```python
from build123d import *

# Parameters (mm, degrees)
BOSS_EXTRUDE1_DEPTH = 76.2
SKETCH2_R           = 2.413
CUT_EXTRUDE1_DEPTH  = 3.175
SKETCH4_R           = 2.413
CUT_EXTRUDE2_DEPTH  = 104.224128115


with BuildPart() as part:
    # Sketch1 → Boss-Extrude1 (new body)
    with BuildSketch(Plane(origin=(0, 0, 0), x_dir=(1, 0, 0), z_dir=(0, 1, 0))):
        Polygon((0, 50.8), (0, 0), (50.8, 0), (50.8, 3.175), (3.175, 3.175), (3.175, 50.8), align=None)
    extrude(amount=BOSS_EXTRUDE1_DEPTH)

    # Sketch2 → Cut-Extrude1 (cut)
    with BuildSketch(Plane(origin=(0, 0, -3.175), x_dir=(-1, 0, 0), z_dir=(0, 0, -1))):
        Polygon((-50.8, 12.7188211), (-6.35, 76.2), (-50.8, 76.2), align=None)
        with Locations((-13.335, 6.35)):
            Circle(SKETCH2_R)
        with Locations((-26.035, 6.35)):
            Circle(SKETCH2_R)
        with Locations((-13.335, 19.05)):
            Circle(SKETCH2_R)
        with Locations((-13.335, 31.75)):
            Circle(SKETCH2_R)
        with Locations((-13.335, 44.45)):
            Circle(SKETCH2_R)
        with Locations((-26.035, 19.05)):
            Circle(SKETCH2_R)
        with Locations((-26.035, 31.75)):
            Circle(SKETCH2_R)
        with Locations((-38.735, 19.05)):
            Circle(SKETCH2_R)
        with Locations((-38.735, 6.35)):
            Circle(SKETCH2_R)
    extrude(amount=-CUT_EXTRUDE1_DEPTH, mode=Mode.SUBTRACT)

    # Sketch4 → Cut-Extrude2 (cut, through all)
    with BuildSketch(Plane(origin=(3.175, 0, 0), x_dir=(0, 0, -1), z_dir=(1, 0, 0))):
        with Locations((27.247845098, 6.35)):
            Circle(SKETCH4_R)
        with Locations((23.960843226, 18.617257994)):
            Circle(SKETCH4_R)
        with Locations((20.673841353, 30.884515988)):
            Circle(SKETCH4_R)
        with Locations((17.38683948, 43.151773982)):
            Circle(SKETCH4_R)
        with Locations((14.099837607, 55.419031975)):
            Circle(SKETCH4_R)
        with Locations((10.812835734, 67.686289969)):
            Circle(SKETCH4_R)
        Polygon((19.05, 76.2), (50.8, 76.2), (50.8, -42.29261314), align=None)
    extrude(amount=-CUT_EXTRUDE2_DEPTH, mode=Mode.SUBTRACT)


solid = part.part
```
Here's how the part is built. I have some questions about the finished solid (model axes, mm). A direction names the side the tool comes from. Coordinates: 2 decimals unless noted, no trailing zeros. Order: outer loops, then holes, each group sorted by start corner. A loop starts at its lowest first (then second) coordinate and runs counter-clockwise, first axis right, second up. Notation, with made-up numbers: M 76,-4 L 101,-4 A16 cw 101,0 Z; hole C 44.25,2.25 d2. An arc over 180 degrees is marked long. Answer as a JSON object with one key per item and string values. Group by question number.
(1) I need wall thicknesses on probe 1 along X at (y, z) = (31, -1); probe 2 along X at (y, z) = (18, -18) (3 decimals); probe 3 along Z at (x, y) = (31, 24) (3 decimals). Which ranges of each line are inside material? Lowest first, please.
(2) If we mould it in two halves opening along Y, with no side actions, what happens to faces 1 (the face through (28.886, 44.015, -1.61)), 2 (the face through (14, 0, -2)), 3 (the face through (19, 29, 0)), 4 (the face through (36.43, 19.77, -1.61))? For each: released by +Y, released by -Y, zero draft, split by the parting line, or undercut.
(3) Suppose I cut it at A-A, the plane y = 44.45. Please give me the cut outline in (x, z) (3 decimals), then the cut area to 3 significant figures.
(4) Suppose I cut it at B-B, the plane y = 6.35. Please give me the cut outline in (x, z) (3 decimals).
(5) Suppose I cut it at D-D, the plane y = 56.5. Please give me the cut outline in (x, z) (1 decimal).
(6) Which directions (+Z, -Z, +X, -X, +Y, -Y) give clear straight access to the entire face, cutting with the end or side of a thin tool? Please do faces 5 (the face through (22, 29, -3.175)), 6 (the face through (1.61, 57.811, -13.786)).
(7) Suppose I cut it at C-C, the plane y = 31.75. Please give me the cut outline in (x, z) (3 decimals).
(8) For pin 1 (12 mm diameter, centred on x = 10.5, y = 68, fed in from -Z) (3 decimals); pin 2 (4.5 mm diameter, centred on x = 26.035, y = 6.35, fed in from -Z); pin 3 (6.5 mm diameter, centred on y = 30.88, z = -20.67, fed in from +X) (3 decimals), each with a flat end and sliding along its axis, tell me the tip position at first contact or that it passes through.
Values found:
{
 "1": {"probe 1": "x = 0 to 11.04, 15.63 to 23.74, 28.33 to 38", "probe 2": "x = 0 to 3.175", "probe 3": "z = -3.175 to 0"},
 "2": {"face 1": "released by +Y", "face 2": "released by -Y", "face 3": "zero draft", "face 4": "undercut"},
 "3": {"outline": "M 0,-27.557 L 3.175,-27.557 L 3.175,-19.421 L 0,-19.421 Z; M 0,-15.353 L 3.175,-15.353 L 3.175,-3.175 L 10.922,-3.175 L 10.922,0 L 0,0 Z; M 15.748,-3.175 L 28.582,-3.175 L 28.582,0 L 15.748,0 Z", "area": "140 mm^2"},
 "4": {"outline": "M 0,-37.766 L 3.175,-37.766 L 3.175,-29.661 L 0,-29.661 Z; M 0,-24.835 L 3.175,-24.835 L 3.175,-3.175 L 10.922,-3.175 L 10.922,0 L 0,0 Z; M 15.748,-3.175 L 23.622,-3.175 L 23.622,0 L 15.748,0 Z; M 28.448,-3.175 L 36.322,-3.175 L 36.322,0 L 28.448,0 Z; M 41.148,-3.175 L 50.8,-3.175 L 50.8,0 L 41.148,0 Z"},
 "5": {"outline": "M 0,-24.3 L 3.2,-24.3 L 3.2,-16.3 L 0,-16.3 Z; M 0,-11.9 L 3.2,-11.9 L 3.2,-3.2 L 20.1,-3.2 L 20.1,0 L 0,0 Z"},
 "6": {"face 5": "-Z, +X, +Y, -Y", "face 6": "+X, -X"},
 "7": {"outline": "M 0,-30.96 L 3.175,-30.96 L 3.175,-22.926 L 0,-22.926 Z; M 0,-18.421 L 3.175,-18.421 L 3.175,-3.175 L 10.922,-3.175 L 10.922,0 L 0,0 Z; M 15.748,-3.175 L 23.622,-3.175 L 23.622,0 L 15.748,0 Z; M 28.448,-3.175 L 37.474,-3.175 L 37.474,0 L 28.448,0 Z"},
 "8": {"pin 1": "stops at z = -3.175", "pin 2": "passes through", "pin 3": "stops at x = 3.175"}
}
